Geometry check sheet. Reference: the model listing, model coordinates, mm. Coordinates: 2 decimals unless noted, no trailing zeros. Write each loop counter-clockwise with the first axis right and the second up, starting at its lowest first coordinate (ties: lowest second). Pieces come first, ordered by that corner, then holes. Notation, with made-up numbers: M -16.5,14 L 37.5,14 A25 cw 37.5,40 Z; hole C -21,-8 d8. An arc over 180 degrees is marked long. Put each result on its own line as item: value. Start each with the question number.
1) Cross-section at B-B on z = 0.6. Record the cut outline in (x, y).
2) Cross-section at D-D on y = -160. Record the cut outline in (x, z).
3) Scan lines: line 1 along Y through (x, z) = (0, 0.6); line 2 along X through (y, z) = (-160, 0.8); line 3 along Y through (x, z) = (-30, -0.55). Record each from-to range of solid material in increasing order.
4) Cross-section at C-C on x = 0. Record the cut outline in (y, z), plus the area to 3 significant figures.
5) Cross-section at A-A on x = -132.5. Record the cut outline in (y, z), plus the area to 3 significant figures.
6) Mould release check, pull along Y, two halves, no side actions. Record for faces 1 (the cylindrical face through (-33.1, 0.1, 0)), 2 (the flat face through (-86, -58, -1.5)), 3 (the cylindrical face through (-248, 14, 0)): released by +Y, released by -Y, zero draft, split by the parting line, or undercut.
from build123d import *

# Parameters (mm, degrees)
SKETCH_R  = 3.1
PAD_DEPTH = 1.5
FILLET_R  = 5


with BuildPart() as part:
    # Sketch → Pad (new body, symmetric)
    with BuildSketch(Plane.XY):
        Polygon((-250, 15), (15, 15), (15, -175), (-15, -175), (-250, -15), align=None)
        Circle(SKETCH_R, mode=Mode.SUBTRACT)
        with Locations((0, -160)):
            Circle(SKETCH_R, mode=Mode.SUBTRACT)
        with Locations((-30, 0)):
            Circle(SKETCH_R, mode=Mode.SUBTRACT)
        with Locations((-235, 0)):
            Circle(SKETCH_R, mode=Mode.SUBTRACT)
        with Locations((-132.5, 0)):
            Circle(SKETCH_R, mode=Mode.SUBTRACT)
        with Locations((0, -80)):
            Circle(SKETCH_R, mode=Mode.SUBTRACT)
    extrude(amount=PAD_DEPTH, both=True)

    # Fillet
    fillet_edges = [part.edges().sort_by_distance(p)[0] for p in [
        (-250, 15, 0),
        (-250, -15, 0),
        (15, 15, 0),
        (-15, -175, 0),
        (15, -175, 0),
    ]]
    fillet(fillet_edges, radius=FILLET_R)


solid = part.part
Answer key:
1. outline: M -250,-12.36 A5 ccw -247.81,-16.49 L -16.27,-174.13 A5 ccw -13.46,-175 L 10,-175 A5 ccw 15,-170 L 15,10 A5 ccw 10,15 L -245,15 A5 ccw -250,10 Z; hole C -235,0 d6.2; hole C -132.5,0 d6.2; hole C -30,0 d6.2; hole C 0,-160 d6.2; hole C 0,-80 d6.2; hole C 0,0 d6.2
2. outline: M -37.03,-1.5 L -3.1,-1.5 L -3.1,1.5 L -37.03,1.5 Z; M 3.1,-1.5 L 15,-1.5 L 15,1.5 L 3.1,1.5 Z
3. line 1: y = -175 to -163.1, -156.9 to -83.1, -76.9 to -3.1, 3.1 to 15
3. line 2: x = -37.03 to -3.1, 3.1 to 15
3. line 3: y = -164.79 to -3.1, 3.1 to 15
4. outline: M -175,-1.5 L -163.1,-1.5 L -163.1,1.5 L -175,1.5 Z; M -156.9,-1.5 L -83.1,-1.5 L -83.1,1.5 L -156.9,1.5 Z; M -76.9,-1.5 L -3.1,-1.5 L -3.1,1.5 L -76.9,1.5 Z; M 3.1,-1.5 L 15,-1.5 L 15,1.5 L 3.1,1.5 Z
4. area: 514 mm²
5. outline: M -95,-1.5 L -3.1,-1.5 L -3.1,1.5 L -95,1.5 Z; M 3.1,-1.5 L 15,-1.5 L 15,1.5 L 3.1,1.5 Z
5. area: 311 mm²
6. face 1: undercut
6. face 2: zero draft
6. face 3: released by +Y
